Autodesk Inventor part; units mm, degrees
ref_plane "YZ Plane" through (0, 0, 0) normal (1, 0, 0) x (0, 1, 0)
ref_plane "XZ Plane" through (0, 0, 0) normal (0, 1, 0) x (-1, 0, 0)
ref_plane "XY Plane" through (0, 0, 0) normal (0, 0, 1) x (1, 0, 0)
sketch "Sketch1" plane through (0, 0, 0) normal (1, 0, 0) x (0, 1, 0)
  line L0 (50, 50) -> (-50, 50)
  line L1 (-50, 50) -> (-50, -50)
  line L2 (-50, -50) -> (50, -50)
  line L3 (50, -50) -> (50, 50)
  line L4 (50, 50) -> (-50, -50) construction
  line L5 (-50, 50) -> (50, -50) construction
  point P0 (0, 0)
  dimension "d0" = 100
  dimension "d1" = 100
extrude "Extrusion1" add sketch "Sketch1" along normal mid plane 10
sketch "Sketch2" plane through (5, 0, 0) normal (1, 0, 0) x (0, 0, -1)
  line L0 (-96.0779, 0) -> (-25, 0) construction
  line L1 (-96.0779, -6) -> (-25, -6)
  line L2 (-25, 6) -> (-96.0779, 6)
  arc A0 (-96.0779, 6) -> (-96.0779, -6) centre (-96.0779, 0) ccw
  arc A1 (-25, -6) -> (-25, 6) centre (-25, 0) ccw
  line L3 (-50, 50) -> (-50, -50)
  point P0 (0, 0)
  point P1 (-60.539, 0)
  point P2 (-50, 6)
  point P3 (-50, -6)
  dimension "d4" = 25
  dimension "d5" = 6
extrude "Extrusion2" cut sketch "Sketch2" along normal through all both and the other way through all contours L3 L2 A1 L1
mirror "Mirror1" about plane through (0, 0, 0) normal (0, 0, 1) of "Extrusion2"
ref_plane "Work Plane1" through (0, 0, 0) normal (0, 0, 1) x (1, 0, 0)
Read the model definition and answer for the solid it produces. Units are mm, in the model's axes. A direction names the side the tool comes from. Coordinates: 2 decimals unless noted, no trailing zeros. Loops run counter-clockwise (first coordinate to the right, second up) from the corner with the lowest first, then second, coordinate; pieces in that order, holes last.
(1) The mould has two halves that part along Y. Classify faces 1 (the face through (0, 6, -38)), 2 (the face through (0, 50, -1)), 3 (the face through (0, 28, 50)): released by +Y, released by -Y, zero draft, split by the parting line, or undercut.
Solution:
face 1: undercut
face 2: released by +Y
face 3: zero draft
(2) Consider line 1 along Y through (x, z) = (-3.5, -27.5); line 2 along Y through (x, z) = (0, -22); line 3 along Z through (x, y) = (0.5, 2). Determine where each line is inside the solid, lowest interval first.
Solution:
line 1: y = -50 to -6, 6 to 50
line 2: y = -50 to -5.2, 5.2 to 50
line 3: z = -19.34 to 19.34
(3) A tool of negligible diameter and unlimited length cuts with its end or side. For faces 4 (the face through (5, -1, 1)), 5 (the face through (0, -6, -37)), 6 (the face through (0, 6, 37)), from which of +Z, -Z, +X, -X, +Y, -Y can it reach the whole face along a straight path? Write none if from no direction.
Solution:
face 4: +Z, -Z, +X, +Y, -Y
face 5: -Z, +X, -X
face 6: +Z, +X, -X
(4) The part is cut by section A-A (z = 28). Determine the outline of the cut face in (x, y).
Solution:
outline: (-5, -50) - (5, -50) - (5, -6) - (-5, -6) - close; (-5, 6) - (5, 6) - (5, 50) - (-5, 50) - close
(5) The part is cut by section C-C (y = 0). Determine the outline of the cut face in (x, z), and give its area (3 significant figures).
Solution:
outline: (-5, -19) - (5, -19) - (5, 19) - (-5, 19) - close
area: 380 mm2
(6) A flat-ended cylindrical pin translates along its axis: pin 1 Ø2 at (x, y) = (1, -0.5) entering from -Z. Find the tip coordinate at first contact, or state that the pin passes through.
Solution:
pin 1: stops at z = -19.19
(7) The part is cut by section B-B (x = -2.5). Determine the outline of the cut face in (y, z), and give its area (3 significant figures).
Solution:
outline: (-50, -50) - (-6, -50) - (-6, -25) arc R6 cw to (6, -25) - (6, -50) - (50, -50) - (50, 50) - (6, 50) - (6, 25) arc R6 cw to (-6, 25) - (-6, 50) - (-50, 50) - close
area: 9,290 mm2
